Check sheet for the drawn part. Datum: minimum x, y, z corner. Units: mm. A direction names the side the tool comes from. Round coordinates to 2 decimals unless told otherwise and drop trailing zeros. Write each loop counter-clockwise with the first axis right and the second up, starting at its lowest first coordinate (ties: lowest second). Pieces come first, ordered by that corner, then holes. Notation, with made-up numbers: (84, -6.5) -> (111, -6.5) arc R29 ccw to (111, 26.5) -> close; hole circle Ø8 at (16.25, 39.5). An arc over 180 degrees is marked (long way). One line per item, written item: value.
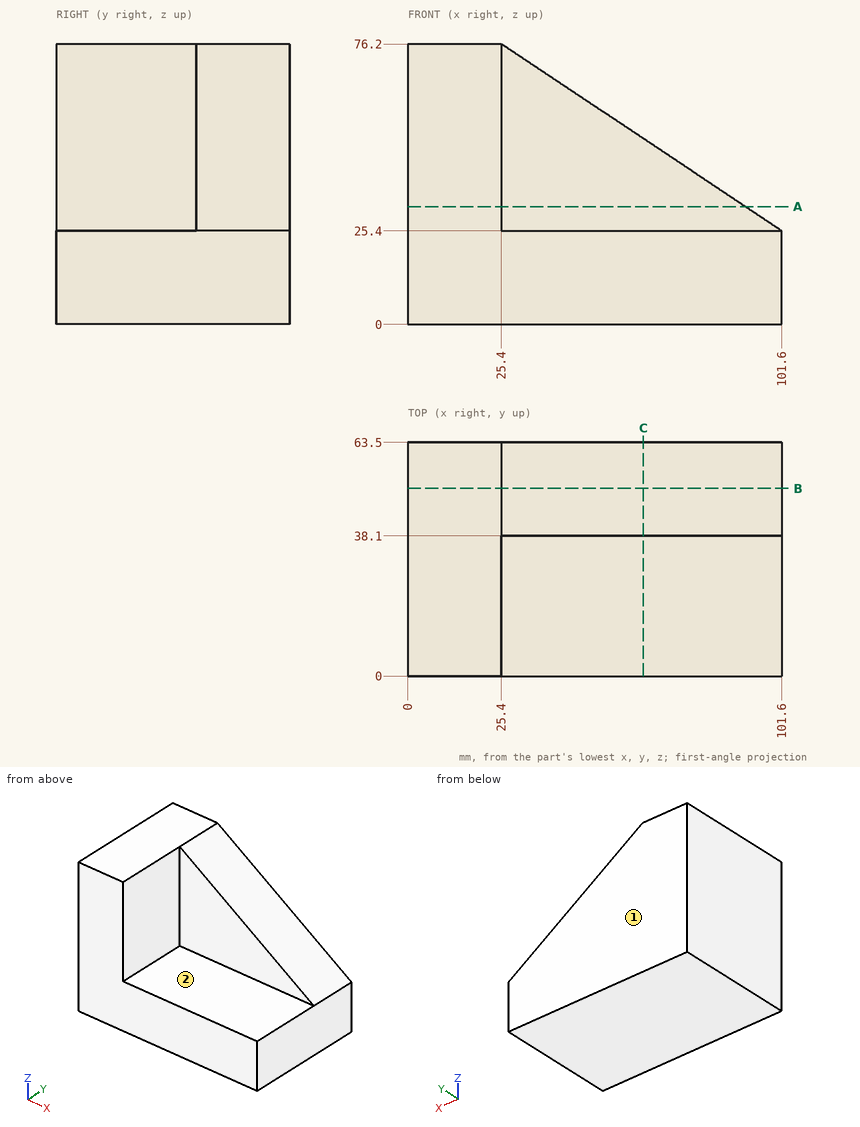
Item 1: Sectioned sample at B-B on y = 51. Enter the section's corners in (x, z), and give its area (3 significant figures).
Answer:
outline: (0, 0) -> (101.6, 0) -> (101.6, 25.4) -> (25.4, 76.2) -> (0, 76.2) -> close
area: 5,810 mm^2
Item 2: Sectioned sample at A-A on z = 32. Enter the section's corners in (x, y), and give its area (3 significant figures).
Answer:
outline: (0, 0) -> (25.4, 0) -> (25.4, 38.1) -> (91.7, 38.1) -> (91.7, 63.5) -> (0, 63.5) -> close
area: 3,300 mm^2
Item 3: Sectioned sample at C-C on x = 64. Enter the section's corners in (y, z), and give its area (3 significant figures).
Answer:
outline: (0, 0) -> (63.5, 0) -> (63.5, 50.47) -> (38.1, 50.47) -> (38.1, 25.4) -> (0, 25.4) -> close
area: 2,250 mm^2
Item 4: Depth check by flat-ended pin: P1, Ø15, axis at x = 50.5, z = 60, coming from the -Y side; P2, Ø6, axis at y = 46, z = 43, coming from the +X side; P3, Ø3, axis at x = 80.5, y = 55.5, coming from the +Z side. Enter the tip coordinate at first touch or a pass-through.
Answer:
P1: stops at y = 38.1
P2: stops at x = 79.7
P3: stops at z = 40.47
Item 5: Thickness scan on line 1 (X direction, y = 13.5, z = 45); line 2 (Y direction, x = 36.5, z = 38). Record the ranges inside material, lowest first.
Answer:
line 1: x = 0 to 25.4
line 2: y = 38.1 to 63.5
Item 6: Tool access check on the marked faces 1 and 2. Record the directions out of +Z, -Z, +X, -X, +Y, -Y that give a thin tool (end or side, any length) a straight path to the whole face; none if there is none.
Answer:
face 1: +Z, -Z, +X, -X, +Y
face 2: +Z, +X, -Y
